Input: part model. Units: mm. Frame: model coordinates. Face numbers are marked on the shaded views. A direction names the side the tool comes from. Coordinates: 2 decimals unless noted, no trailing zeros. Loops run counter-clockwise (first coordinate to the right, second up) from the corner with the lowest first, then second, coordinate; pieces in that order, holes last.
(1) Line query: L1, parallel to X at y = 4.5, z = 6.5; L2, parallel to Z at x = -17.95, y = 6; L3, parallel to X at y = 8.25, z = -10. Output: solid intervals per line, ascending.
(2) Section C-C, the plane z = -16. Return loops of the section in (x, y).
(3) Set-up query: the marked faces 1, 2, 3, 4 and 5. Return all of +Z, -Z, +X, -X, +Y, -Y with unobstructed straight access to the full face (end or side cutting, diameter ignored); none if empty.
(4) Section A-A, the plane z = -9.5. Return loops of the section in (x, y), then the cut area to 3 significant figures.
(5) Section B-B, the plane x = 31.5. Return loops of the section in (y, z), then the cut area to 3 significant figures.
(6) Contact query for flat-ended pins moving along their axis: P1, Ø2.5, axis at y = 11, z = -23, coming from the -X side; P2, Ø3, axis at x = -17.5, z = 20.5, coming from the -Y side; P3, Ø5, axis at x = -17.95, z = -24, coming from the +Y side; P4, Ø5, axis at y = 11, z = -17, coming from the +X side. Output: stop coordinate, or through.
(7) Section D-D, the plane x = 8.05. Return loops of the section in (y, z).
(8) Mould query, pull axis Z, two halves, no side actions, for the marked faces 6, 7 and 8. Classes: released by +Z, released by -Z, zero draft, split by the parting line, or undercut.
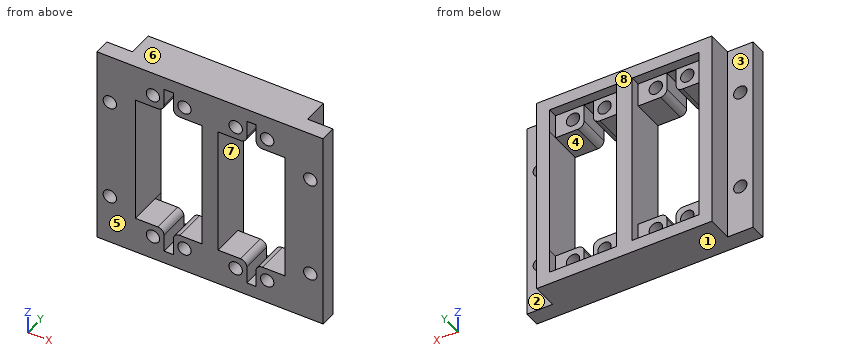
```python
from build123d import *

# Parameters (mm, degrees)
SKETCH2_W           = 55
SKETCH2_H           = 63
SKETCH2_R           = 2.1
BOSS_EXTRUDE1_DEPTH = 13
SKETCH3_W           = 20.991665644
SKETCH3_H           = 7.5
CUT_EXTRUDE1_DEPTH  = 3
SKETCH2_3_W         = 8
SKETCH2_3_H         = 63
SKETCH2_3_R         = 2.1
BOSS_EXTRUDE2_DEPTH = 5


with BuildPart() as part:
    # Sketch2 → Boss-Extrude1 (new body)
    with BuildSketch(Plane(origin=(0, 0, 0), x_dir=(1, 0, 0), z_dir=(0, 1, 0))):
        Rectangle(SKETCH2_W, SKETCH2_H)
        with Locations((8.05, 24)):
            Circle(SKETCH2_R, mode=Mode.SUBTRACT)
        with Locations((17.95, 24)):
            Circle(SKETCH2_R, mode=Mode.SUBTRACT)
        with Locations((8.05, -24)):
            Circle(SKETCH2_R, mode=Mode.SUBTRACT)
        with Locations((17.95, -24)):
            Circle(SKETCH2_R, mode=Mode.SUBTRACT)
        with Locations((-8.05, 24)):
            Circle(SKETCH2_R, mode=Mode.SUBTRACT)
        with Locations((-17.95, 24)):
            Circle(SKETCH2_R, mode=Mode.SUBTRACT)
        with Locations((-8.05, -24)):
            Circle(SKETCH2_R, mode=Mode.SUBTRACT)
        with Locations((-17.95, -24)):
            Circle(SKETCH2_R, mode=Mode.SUBTRACT)
        with BuildLine():
            Line((16.45, 20.1), (23.5, 20.1))
            Line((23.5, 20.1), (23.5, -20.1))
            Line((23.5, -20.1), (16.45, -20.1))
            ThreePointArc((16.45, -20.1), (15.035786438, -20.685786438), (14.45, -22.1))
            Line((14.45, -22.1), (14.45, -27.5))
            Line((14.45, -27.5), (11.55, -27.5))
            Line((11.55, -27.5), (11.55, -22.1))
            ThreePointArc((11.55, -22.1), (10.964213562, -20.685786438), (9.55, -20.1))
            Line((9.55, -20.1), (2.5, -20.1))
            Line((2.5, -20.1), (2.5, 20.1))
            Line((2.5, 20.1), (9.55, 20.1))
            ThreePointArc((9.55, 20.1), (10.964213562, 20.685786438), (11.55, 22.1))
            Line((11.55, 22.1), (11.55, 27.5))
            Line((11.55, 27.5), (14.45, 27.5))
            Line((14.45, 27.5), (14.45, 22.1))
            ThreePointArc((14.45, 22.1), (15.035786438, 20.685786438), (16.45, 20.1))
        make_face(mode=Mode.SUBTRACT)
        with BuildLine():
            Line((-16.45, 20.1), (-23.5, 20.1))
            Line((-23.5, 20.1), (-23.5, -20.1))
            Line((-23.5, -20.1), (-16.45, -20.1))
            ThreePointArc((-16.45, -20.1), (-15.035786438, -20.685786438), (-14.45, -22.1))
            Line((-14.45, -22.1), (-14.45, -27.5))
            Line((-14.45, -27.5), (-11.55, -27.5))
            Line((-11.55, -27.5), (-11.55, -22.1))
            ThreePointArc((-11.55, -22.1), (-10.964213562, -20.685786438), (-9.55, -20.1))
            Line((-9.55, -20.1), (-2.5, -20.1))
            Line((-2.5, -20.1), (-2.5, 20.1))
            Line((-2.5, 20.1), (-9.55, 20.1))
            ThreePointArc((-9.55, 20.1), (-10.964213562, 20.685786438), (-11.55, 22.1))
            Line((-11.55, 22.1), (-11.55, 27.5))
            Line((-11.55, 27.5), (-14.45, 27.5))
            Line((-14.45, 27.5), (-14.45, 22.1))
            ThreePointArc((-14.45, 22.1), (-15.035786438, 20.685786438), (-16.45, 20.1))
        make_face(mode=Mode.SUBTRACT)
    extrude(amount=BOSS_EXTRUDE1_DEPTH)

    # Sketch3 → Cut-Extrude1 (cut)
    with BuildSketch(Plane(origin=(0, 13, 0), x_dir=(1, 0, 0), z_dir=(0, 1, 0))):
        with Locations((12.995832822, 23.85)):
            Rectangle(SKETCH3_W, SKETCH3_H)
        with Locations((12.995832822, -23.85)):
            Rectangle(SKETCH3_W, SKETCH3_H)
        with Locations((-12.995832822, -23.85)):
            Rectangle(SKETCH3_W, SKETCH3_H)
        with Locations((-12.995832822, 23.85)):
            Rectangle(SKETCH3_W, SKETCH3_H)
    extrude(amount=-CUT_EXTRUDE1_DEPTH, mode=Mode.SUBTRACT)

    # Sketch2_3 → Boss-Extrude2 (add)
    with BuildSketch(Plane(origin=(0, 0, 0), x_dir=(1, 0, 0), z_dir=(0, 1, 0))):
        with Locations((-31.5, 0)):
            Rectangle(SKETCH2_3_W, SKETCH2_3_H)
        with Locations((-31.5, -16)):
            Circle(SKETCH2_3_R, mode=Mode.SUBTRACT)
        with Locations((-31.5, 16)):
            Circle(SKETCH2_3_R, mode=Mode.SUBTRACT)
        with Locations((31.5, 0)):
            Rectangle(SKETCH2_3_W, SKETCH2_3_H)
        with Locations((31.5, 16)):
            Circle(SKETCH2_3_R, mode=Mode.SUBTRACT)
        with Locations((31.5, -16)):
            Circle(SKETCH2_3_R, mode=Mode.SUBTRACT)
    extrude(amount=BOSS_EXTRUDE2_DEPTH)


solid = part.part
```
Report:
1. L1: x = -35.5 to -23.5, -2.5 to 2.5, 23.5 to 35.5
1. L2: z = -31.5 to -26.1, -21.9 to -20.1, 20.1 to 21.9, 26.1 to 31.5
1. L3: x = -27.5 to -23.5, -2.5 to 2.5, 23.5 to 27.5
2. outline: (-35.5, 0) - (-33.6, 0) - (-33.6, 5) - (-35.5, 5) - close; (-29.4, 0) - (-23.5, 0) - (-23.5, 13) - (-27.5, 13) - (-27.5, 5) - (-29.4, 5) - close; (-2.5, 0) - (2.5, 0) - (2.5, 13) - (-2.5, 13) - close; (23.5, 0) - (29.4, 0) - (29.4, 5) - (27.5, 5) - (27.5, 13) - (23.5, 13) - close; (33.6, 0) - (35.5, 0) - (35.5, 5) - (33.6, 5) - close
3. face 1: -Z, +X, -X, +Y, -Y
3. face 2: +Z, -Z, +X, +Y
3. face 3: +Z, -Z, -X, +Y
3. face 4: +Y, -Y
3. face 5: +Z, -Z, +X, -X, -Y
4. outline: (-35.5, 0) - (-23.5, 0) - (-23.5, 13) - (-27.5, 13) - (-27.5, 5) - (-35.5, 5) - close; (-2.5, 0) - (2.5, 0) - (2.5, 13) - (-2.5, 13) - close; (23.5, 0) - (35.5, 0) - (35.5, 5) - (27.5, 5) - (27.5, 13) - (23.5, 13) - close
4. area: 249 mm2
5. outline: (0, -31.5) - (5, -31.5) - (5, -18.1) - (0, -18.1) - close; (0, -13.9) - (5, -13.9) - (5, 13.9) - (0, 13.9) - close; (0, 18.1) - (5, 18.1) - (5, 31.5) - (0, 31.5) - close
5. area: 273 mm2
6. P1: stops at x = -27.5
6. P2: stops at y = 0
6. P3: stops at y = 10
6. P4: stops at x = 27.5
7. outline: (0, -31.5) - (13, -31.5) - (13, -27.6) - (10, -27.6) - (10, -26.1) - (0, -26.1) - close; (0, -21.9) - (10, -21.9) - (10, -20.1) - (0, -20.1) - close; (0, 20.1) - (10, 20.1) - (10, 21.9) - (0, 21.9) - close; (0, 26.1) - (10, 26.1) - (10, 27.6) - (13, 27.6) - (13, 31.5) - (0, 31.5) - close
8. face 6: released by +Z
8. face 7: undercut
8. face 8: zero draft
